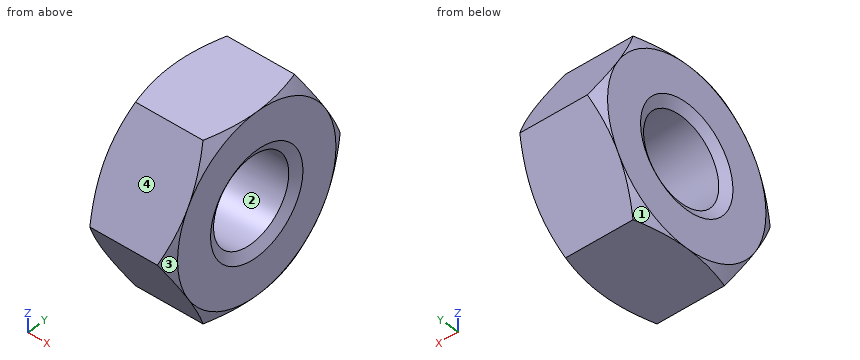
Autodesk Inventor part; units mm, degrees
ref_plane "Work Plane1" through (-6.7833, 0, 0) normal (0, -0.8660254, -0.5) x (1, 0, 0)
ref_plane "YZ Plane" through (0, 0, 0) normal (1, 0, 0) x (0, 1, 0)
ref_plane "XZ Plane" through (0, 0, 0) normal (0, 1, 0) x (-1, 0, 0)
sketch "Эскиз1" plane through (0, 0, 0) normal (1, 0, 0) x (0, 1, 0)
  line L0 (-3.4641, 0) -> (-1.7321, 3)
  line L1 (-1.7321, 3) -> (1.7321, 3)
  line L2 (1.7321, 3) -> (3.4641, 0)
  line L3 (3.4641, 0) -> (1.7321, -3)
  line L4 (1.7321, -3) -> (-1.7321, -3)
  line L5 (-1.7321, -3) -> (-3.4641, 0)
  point P0 (0, 0)
  point P1 (0, 0)
  dimension "d0" = 6.9282
extrude "Базовый элемент" add sketch "Эскиз1" along normal blind 2.8
sketch "Эскиз2" plane through (0, 0, 0) normal (0, 0, 1) x (1, 0, 0)
  line L0 (0, 1.7321) -> (0, 3.4641)
  line L1 (0, 3.4641) -> (2.8, 3.4641)
  line L2 (2.8, 1.7321) -> (2.8, 3.4641)
  line L3 (-0.56, 0) -> (3.36, 0)
  line L4 (0.2679, 3.4641) -> (0, 3)
  line L5 (2.5321, 3.4641) -> (2.8, 3)
  dimension "d3" = 30
  dimension "d4" = 30
  dimension "d5" = 6
  dimension "d6" = 6
revolve "Фаска1" cut sketch "Эскиз2" angle 360 about axis through (-10, 0, 0) along (1, 0, 0)
sketch "Эскиз3" plane through (2.8, 0, 0) normal (1, 0, 0) x (0, 0, -1)
  arc A0 (-1.5, -2.5981) -> (1.5, -2.5981) centre (0, 0) ccw
hole "Резьба" at (2.8, 0, 0) direction (-1, 0, 0) diameter 2.85 end through all
chamfer "Фаска2" distance 0.3248 angle 30 1 edges at (2.8, 0, 1.425) measured on face at (2.8, -2.4606, -0.0573)
chamfer "Фаска3" distance 0.3248 angle 30 1 edges at (0, 0, 1.425) measured on face at (0, -2.4606, -0.0573)
ref_plane "Work Plane1" through (-6.7833, 0, 0) normal (0, -0.8660254, -0.5) x (1, 0, 0)
equation "\"d0\" = 1.1547 * SW"
equation "\"d1\" = KOH"
equation "\"d3\" = ANG1"
equation "\"d4\" = ANG2"
equation "\"d5\" = SW0"
equation "\"d6\" = SW01"
equation "\"d8\" = -0.5 * GD1 + 0.5 * NND"
equation "\"d40\" = -0.5 * GD1 + 0.5 * NND"
equation "\"d10\" = -0.5 * GD1 + 0.5 * NND"
equation "\"d41\" = -0.5 * GD1 + 0.5 * NND"
equation "\"ANG1\" = 30deg"
equation "\"ANG2\" = 30deg"
equation "\"NND\" = 3.5"
equation "\"KOH\" = 2.8"
equation "\"SW\" = 6"
equation "\"SW0\" = SW"
equation "\"SW01\" = SW"
equation "\"GUL\" = 0.541266 * PTC"
equation "\"WFT\" = 0"
equation "\"THREADDIA\" = 3.5"
equation "\"TOA\" = 30deg"
equation "\"PTC\" = 0.6"
equation "\"E0\" = 1.155 * SW"
equation "\"GAL\" = 0.541266 * PTC"
properties part number "AS 1112 - M3,5  Тип 10" material "Сталь, мягкая"
Can you work these out from the model? Positions are in its coordinate system, mm. Face numbers are marked on the shaded views. Coordinates: 2 decimals unless noted, no trailing zeros. Order: outer loops, then holes, each group sorted by start corner. A loop starts at its lowest first (then second) coordinate and runs counter-clockwise, first axis right, second up. Notation, with made-up numbers: (24, 1) -> (58, 1) arc R3 ccw to (58, 6) -> close; hole circle Ø3 at (48.25, -36.5). An arc over 180 degrees is marked (long way). Use one line per item in the form item = value.
Q1. I need wall thicknesses on L1, parallel to Z at x = 1.9, y = 0 (3 decimals); L2, parallel to Z at x = 0.5, y = -0.5; L3, parallel to Y at x = 1.5, z = -0.25. Which ranges of each line are inside material? Lowest first, please.
From the geometry:
L1 = -3 to -1.425, 1.425 to 3
L2 = -3 to -1.33, 1.33 to 3
L3 = -3.32 to -1.4, 1.4 to 3.32
Q2. Imagine slicing it at A-A, the plane x = 0.7. List the corners of the cut face in (y, z) for me (3 decimals).
From the geometry:
outline = (-3.464, 0) -> (-1.732, -3) -> (1.732, -3) -> (3.464, 0) -> (1.732, 3) -> (-1.732, 3) -> close; hole circle Ø2.85 at (0, 0)
Q3. We'd pull the mould along Z, two halves only. Please class the marked faces 1, 2, 3 and 4: released by +Z, released by -Z, zero draft, split by the parting line, or undercut.
From the geometry:
face_1 = released by -Z
face_2 = undercut
face_3 = split by the parting line
face_4 = released by +Z
